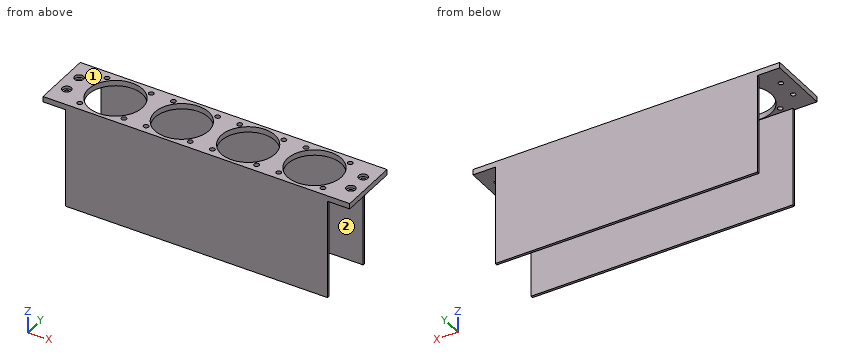
Autodesk Fusion 360 part; units mm, degrees
sketch "Sketch1" plane through (0, 0, 0) normal (0, 0, 1) x (1, 0, 0)
  line L0 (-111, 0.4) -> (111, 0.4)
  line L1 (111, 0.4) -> (111, 44.05)
  line L2 (111, 44.05) -> (-111, 44.05)
  line L3 (-111, 44.05) -> (-111, 0.4)
extrude "Extrude1" add sketch "Sketch1" along normal blind 4
sketch "Sketch2" plane through (0, 0, 0) normal (0, 0, 1) x (1, 0, 0)
  circle A0 centre (-72, 22.225) radius 19.5
  circle A1 centre (-88, 6.225) radius 1.8
  circle A2 centre (-88, 38.225) radius 1.8
  circle A3 centre (-56, 6.225) radius 1.8
  circle A4 centre (-56, 38.225) radius 1.8
  circle A5 centre (-24, 22.225) radius 19.5
  circle A6 centre (-40, 6.225) radius 1.8
  circle A7 centre (-40, 38.225) radius 1.8
  circle A8 centre (-8, 6.225) radius 1.8
  circle A9 centre (-8, 38.225) radius 1.8
  circle A10 centre (24, 22.225) radius 19.5
  circle A11 centre (8, 6.225) radius 1.8
  circle A12 centre (8, 38.225) radius 1.8
  circle A13 centre (40, 6.225) radius 1.8
  circle A14 centre (40, 38.225) radius 1.8
  circle A15 centre (72, 22.225) radius 19.5
  circle A16 centre (56, 6.225) radius 1.8
  circle A17 centre (56, 38.225) radius 1.8
  circle A18 centre (88, 6.225) radius 1.8
  circle A19 centre (88, 38.225) radius 1.8
  circle A20 centre (-102.82, 15) radius 1.7
  circle A21 centre (-102.82, 29.45) radius 1.7
  circle A22 centre (102.82, 15) radius 1.7
  circle A23 centre (102.82, 29.45) radius 1.7
extrude "Extrude2" cut sketch "Sketch2" along normal blind 4
sketch "Sketch3" plane through (0, 0, 0) normal (0, 0, 1) x (1, 0, 0)
  line L0 (-94.8, 42.25) -> (94.8, 42.25)
  line L1 (94.8, 42.25) -> (94.8, 44.05)
  line L2 (94.8, 44.05) -> (-94.8, 44.05)
  line L3 (-94.8, 44.05) -> (-94.8, 42.25)
  line L4 (-94.8, 0.4) -> (94.8, 0.4)
  line L5 (94.8, 0.4) -> (94.8, 2.2)
  line L6 (94.8, 2.2) -> (-94.8, 2.2)
  line L7 (-94.8, 2.2) -> (-94.8, 0.4)
extrude "Extrude3" add sketch "Sketch3" against normal blind 72
ref_plane "WorkPlane1" through (0, 0, 4) normal (0, 0, 1) x (1, 0, 0)
sketch "Sketch4" plane through (0, 0, 4) normal (0, 0, 1) x (1, 0, 0)
  circle A0 centre (-102.82, 15) radius 3.25
  circle A1 centre (-102.82, 29.45) radius 3.25
  circle A2 centre (102.82, 15) radius 3.25
  circle A3 centre (102.82, 29.45) radius 3.25
extrude "Extrude4" cut sketch "Sketch4" against normal blind 2
Build history of the part. All positions in model axes, mm. Face numbers are marked on the shaded views. A direction names the side the tool comes from. Round coordinates to 2 decimals unless told otherwise and drop trailing zeros. Write each loop counter-clockwise with the first axis right and the second up, starting at its lowest first coordinate (ties: lowest second). Pieces come first, ordered by that corner, then holes. Notation, with made-up numbers: (8, -38.5) - (26, -38.5) arc R37 ccw to (26, -2.5) - close; hole circle Ø9 at (-1.5, 46.5). An arc over 180 degrees is marked (long way). Write each question's results on one line, items separated by ' | '. Start each with the question number.
Item 1: Saw through at A-A (x = -72). Write the cut outline in (y, z) (3 decimals), and give its area (3 significant figures).
Item 2: Which spindle directions (+Z, -Z, +X, -X, +Y, -Y) get a long thin tool onto all of the face, cutting with end or side? Do the marked faces 1 and 2. Say none if no direction does.
Item 3: Drop flat-ended pins along their axis: P1, Ø4, axis at x = 40, y = 6.225, coming from the -Z side; P2, Ø0.9, axis at y = 43.5, z = -46, coming from the +X side; P3, Ø4, axis at x = 102.82, y = 15, coming from the +Z side. Give the stop position or say it passes through.
Item 4: Saw through at D-D (x = 81.5). Write the cut outline in (y, z).
Item 5: Saw through at C-C (x = 1.5). Write the cut outline in (y, z), and give its area (3 significant figures).
Item 6: Wall check: L1, parallel to X at y = 22.5, z = 1; L2, parallel to Y at x = 3, z = -5; L3, parallel to Y at x = 56, z = 2 (3 decimals). Give the ranges that are in metal, low to high. Write a range as [from, to].
Item 7: Saw through at B-B (z = -63). Write the cut outline in (x, y).
Results are:
1) outline: (0.4, -72) - (2.2, -72) - (2.2, 0) - (2.725, 0) - (2.725, 4) - (0.4, 4) - close; (41.725, 0) - (42.25, 0) - (42.25, -72) - (44.05, -72) - (44.05, 4) - (41.725, 4) - close | area: 278 mm²
2) face 1: +Z, +X, -X, +Y, -Y | face 2: -Z, +X, -X
3) P1: stops at z = 0 | P2: stops at x = 94.8 | P3: stops at z = 2
4) outline: (0.4, -72) - (2.2, -72) - (2.2, 0) - (5.2, 0) - (5.2, 4) - (0.4, 4) - close; (39.25, 0) - (42.25, 0) - (42.25, -72) - (44.05, -72) - (44.05, 4) - (39.25, 4) - close
5) outline: (0.4, -72) - (2.2, -72) - (2.2, 0) - (42.25, 0) - (42.25, -72) - (44.05, -72) - (44.05, 4) - (0.4, 4) - close | area: 434 mm²
6) L1: x = [-111, -91.5], [-52.5, -43.5], [-4.5, 4.5], [43.5, 52.5], [91.5, 111] | L2: y = [0.4, 2.2], [42.25, 44.05] | L3: y = [0.4, 4.425], [8.025, 11.078], [33.372, 36.425], [40.025, 44.05]
7) outline: (-94.8, 0.4) - (94.8, 0.4) - (94.8, 2.2) - (-94.8, 2.2) - close; (-94.8, 42.25) - (94.8, 42.25) - (94.8, 44.05) - (-94.8, 44.05) - close
